Read the model definition and answer for the solid it produces. Units are mm, in the model's axes. A direction names the side the tool comes from. Round coordinates to 2 decimals unless told otherwise and drop trailing zeros. Order: outer loops, then holes, each group sorted by start corner. A loop starts at its lowest first (then second) coordinate and runs counter-clockwise, first axis right, second up. Notation, with made-up numbers: (74.5, -24) - (121.5, -24) arc R20 cw to (121.5, 4) - close; hole circle Ø3 at (66.5, 73). An arc over 180 degrees is marked (long way). Put each result on its own line as item: value. Start each with the question number.
Q1. Which of the six approach directions +Z, -Z, +X, -X, +Y, -Y give full straight-line access (tool end or side, diameter ignored) to faces 1 (the face through (25, -25, -76.2)), 2 (the face through (12.7, -31, -45)), 3 (the face through (6, -25, -25.4)), 4 (the face through (27, -12, 0)), 5 (the face through (38.894, -25, -13))?
Q2. Find the intervals of material crossed by line 1 along X through (y, z) = (-32, -28.5); line 2 along X through (y, z) = (-30.5, -18); line 3 along Y through (x, z) = (14, -39), in increasing order. Write a range as from..to.
Q3. Each of these flat-tipped pins is pushed along its axis until it touches: pin 1 Ø6.5 at (y, z) = (-3.5, -17) entering from -X; pin 2 Ø2 at (y, z) = (-43.5, -17) entering from +X; pin 3 Ø8 at (x, y) = (27, -29) entering from +Z. Where does it stop, or does it pass through?
Q4. Section A-A on y = -25 is taken. Give the vertices of the cut face in (x, z), then the cut area to 3 significant figures.
Q5. Section C-C on x = 15.5 is taken. Give the vertices of the cut face in (y, z).
Q6. Section B-B on z = -6.5 is taken. Give the vertices of the cut face in (x, y).
Q7. Section D-D on z = -35 is taken. Give the vertices of the cut face in (x, y).
Q8. For a pull along X with two mould halves and no side action, classify faces 6 (the face through (25, -31, -63.5)), 7 (the face through (50.8, -25, -51)), 8 (the face through (38.1, -31, -32)), 9 (the face through (25, 0, -46)) as pulls with the +X half, pulls with the -X half, needs draft (parallel to the pull), parting line crosses it, or undercut.
from build123d import *

# Parameters (mm, degrees)
F0_W     = 50.8
F0_H     = 76.2
F1_DEPTH = 50.8
F2_T     = -12.7
F3_W     = 12.7
F3_H     = 25.4
F4_DEPTH = 79.708762


with BuildPart() as f1:
    # F0 (on Front) → F1 (new body)
    with BuildSketch(Plane.XZ):
        with Locations((25.4, -38.1)):
            Rectangle(F0_W, F0_H)
    extrude(amount=F1_DEPTH)

    # F2
    f2_openings = [f1.faces().sort_by_distance(p)[0] for p in [
        (25.4, -50.8, -38.1),
        (25.4, -25.4, 0),
    ]]
    offset(amount=F2_T, openings=f2_openings)

    # F3 (on Front) → F4 (cut)
    with BuildSketch(Plane.XZ):
        with Locations((6.35, -12.7)):
            Rectangle(F3_W, F3_H)
        with Locations((45.243796, -12.7)):
            Rectangle(F3_W, F3_H)
    extrude(amount=F4_DEPTH, mode=Mode.SUBTRACT)


solid = f1.part
Findings:
1. face 1: -Z, +X, -X, +Y, -Y
1. face 2: +Z, -Y
1. face 3: +Z, -X, +Y, -Y
1. face 4: +Z, +X, -X, +Y, -Y
1. face 5: +Z, +X, +Y, -Y
2. line 1: 0..12.7, 38.1..50.8
2. line 2: 38.1..38.89
2. line 3: -12.7..0
3. pin 1: x = 12.7
3. pin 2: x = 38.89
3. pin 3: z = -63.5
4. outline: (0, -76.2) - (50.8, -76.2) - (50.8, -25.4) - (38.89, -25.4) - (38.89, 0) - (38.1, 0) - (38.1, -63.5) - (12.7, -63.5) - (12.7, -25.4) - (0, -25.4) - close
4. area: 1,630 mm2
5. outline: (-50.8, -76.2) - (0, -76.2) - (0, 0) - (-12.7, 0) - (-12.7, -63.5) - (-50.8, -63.5) - close
6. outline: (12.7, -12.7) - (38.1, -12.7) - (38.1, -50.8) - (38.89, -50.8) - (38.89, 0) - (12.7, 0) - close
7. outline: (0, -50.8) - (12.7, -50.8) - (12.7, -12.7) - (38.1, -12.7) - (38.1, -50.8) - (50.8, -50.8) - (50.8, 0) - (0, 0) - close
8. face 6: undercut
8. face 7: pulls with the +X half
8. face 8: undercut
8. face 9: needs draft
